from build123d import *

# Parameters (mm, degrees)
SKETCH1_R           = 12.5
SKETCH1_R_2         = 9
BOSS_EXTRUDE1_DEPTH = 80
SKETCH2_R           = 3.5
BOSS_EXTRUDE2_DEPTH = 5


with BuildPart() as part:
    # Sketch1 → Boss-Extrude1 (new body)
    with BuildSketch(Plane.XY):
        Circle(SKETCH1_R)
        Circle(SKETCH1_R_2, mode=Mode.SUBTRACT)
    extrude(amount=BOSS_EXTRUDE1_DEPTH)

    # Sketch2 → Boss-Extrude2 (add, symmetric)
    with BuildSketch(Plane(origin=(0, 0, 0), x_dir=(1, 0, 0), z_dir=(0, 1, 0))):
        with BuildLine():
            Line((-12.5, 0), (12.5, 0))
            Line((12.5, 0), (12.5, 12))
            ThreePointArc((12.5, 12), (0, 24.5), (-12.5, 12))
            Line((-12.5, 12), (-12.5, 0))
        make_face()
        with Locations((0, 13)):
            Circle(SKETCH2_R, mode=Mode.SUBTRACT)
    extrude(amount=BOSS_EXTRUDE2_DEPTH, both=True)


solid = part.part
Work out the finished part from the listing and answer in its coordinate system (mm). A direction names the side the tool comes from. Round coordinates to 2 decimals unless told otherwise and drop trailing zeros. Write each loop counter-clockwise with the first axis right and the second up, starting at its lowest first coordinate (ties: lowest second). Pieces come first, ordered by that corner, then holes.
1) A cutting plane is placed at B-B (z = -13). Give the vertices of the cut face in (x, y).
2) A cutting plane is placed at C-C (y = 7.75). Give the vertices of the cut face in (x, z), plus the area to 3 significant figures.
3) A cutting plane is placed at A-A (x = 0). Give the vertices of the cut face in (y, z).
4) A tool of negligible diameter and unlimited length cuts with its end or side. For faces 1 (the flat face through (3, -5, -10)), 2 (the flat face through (-12.5, 0, -6)), 3 (the cylindrical face through (0.275, 0.07, -24.497)), 4 (the flat face through (0, 10, 0)), 5 (the cylindrical face through (-1.172, 8.923, 39.44)), from which of +Z, -Z, +X, -X, +Y, -Y can it reach the whole face along a straight path? Write none if from no direction.
5) Straight lines are drawn through the part: line 1 (Z direction, x = 0, y = -0.5); line 2 (Y direction, x = 0, z = 40); line 3 (Y direction, x = -3, z = -16). For each, find the intervals that lie inside material, in ascending order.
6) Given pin 1 Ø12 at (x, z) = (-2, -7.5) entering from +Y; pin 2 Ø4 at (x, y) = (2, -3) entering from -Z; pin 3 Ø1.5 at (x, z) = (-6.5, -13.5) entering from -Y; pin 4 Ø4 at (x, z) = (7.5, 62.5) entering from -Y (3 decimals), each flat-ended and moving along its own axis, determine where each tip first touches the part or whether it passes through.
7) The mould has two halves that part along X. Classify faces 6 (the flat face through (3, 5, -10)), 7 (the cylindrical face through (-0.759, -0.07, -9.583)), 8 (the flat face through (0, 0, 0)), 9 (the flat face through (12.5, 0, -6)): pulls with the +X half, pulls with the -X half, needs draft (parallel to the pull), parting line crosses it, or undercut.
8) A cutting plane is placed at D-D (y = -2.75). Give the vertices of the cut face in (x, z).
Completed:
1. outline: (-12.46, -5) - (-3.5, -5) - (-3.5, 5) - (-12.46, 5) - close; (3.5, -5) - (12.46, -5) - (12.46, 5) - (3.5, 5) - close
2. outline: (-9.81, 0) - (-4.58, 0) - (-4.58, 80) - (-9.81, 80) - close; (4.58, 0) - (9.81, 0) - (9.81, 80) - (4.58, 80) - close
2. area: 837 mm2
3. outline: (-12.5, 0) - (-9, 0) - (-9, 80) - (-12.5, 80) - close; (-5, -24.5) - (5, -24.5) - (5, -16.5) - (-5, -16.5) - close; (-5, -9.5) - (5, -9.5) - (5, 0) - (-5, 0) - close; (9, 0) - (12.5, 0) - (12.5, 80) - (9, 80) - close
4. face 1: -Z, +X, -X, -Y
4. face 2: +Z, -Z, -X, +Y, -Y
4. face 3: -Z, +Y, -Y
4. face 4: -Z, +X, -X, +Y
4. face 5: +Z
5. line 1: z = -24.5 to -16.5, -9.5 to 0
5. line 2: y = -12.5 to -9, 9 to 12.5
5. line 3: y = -5 to 5
6. pin 1: stops at y = 5
6. pin 2: stops at z = -24.5
6. pin 3: stops at y = -5
6. pin 4: stops at y = -11.225
7. face 6: needs draft
7. face 7: undercut
7. face 8: undercut
7. face 9: pulls with the +X half
8. outline: (-12.5, -12) arc R12.5 ccw to (12.5, -12) - (12.5, 0) - (12.19, 0) - (12.19, 80) - (8.57, 80) - (8.57, 0) - (-8.57, 0) - (-8.57, 80) - (-12.19, 80) - (-12.19, 0) - (-12.5, 0) - close; hole circle Ø7 at (0, -13)
